Design review of the part built by this model. Coordinates are the model's own, in mm. Round coordinates to 2 decimals unless told otherwise and drop trailing zeros. Order: outer loops, then holes, each group sorted by start corner. A loop starts at its lowest first (then second) coordinate and runs counter-clockwise, first axis right, second up. Notation, with made-up numbers: M -37.5,40 L 9.5,40 A37 ccw 9.5,79 Z; hole C 20.25,38.5 d6. An arc over 180 degrees is marked long. Write item = value, one per line. Start each with the question number.
```python
from build123d import *

# Parameters (mm, degrees)
SKETCH_1_W      = 70.5
SKETCH_1_H      = 100.35
SKETCH_1_R      = 1.5
EXTRUDE_1_DEPTH = 1.6
FILLET_1_R      = 10


with BuildPart() as part:
    # 草圖1 → 填料-伸長1 (new body)
    with BuildSketch(Plane(origin=(0, 0, 0), x_dir=(1, 0, 0), z_dir=(0, 1, 0))):
        Rectangle(SKETCH_1_W, SKETCH_1_H)
        with Locations((-30, 35)):
            Circle(SKETCH_1_R, mode=Mode.SUBTRACT)
        with Locations((30, 35)):
            Circle(SKETCH_1_R, mode=Mode.SUBTRACT)
        with Locations((-30, -35)):
            Circle(SKETCH_1_R, mode=Mode.SUBTRACT)
        with Locations((30, -35)):
            Circle(SKETCH_1_R, mode=Mode.SUBTRACT)
        with BuildLine():
            Line((-25.5, 1.5), (25.5, 1.5))
            ThreePointArc((25.5, 1.5), (27, 0), (25.5, -1.5))
            Line((25.5, -1.5), (-25.5, -1.5))
            ThreePointArc((-25.5, -1.5), (-27, 0), (-25.5, 1.5))
        make_face(mode=Mode.SUBTRACT)
        with BuildLine():
            Line((1.5, 40.5), (1.5, 6.5))
            ThreePointArc((1.5, 6.5), (0, 5), (-1.5, 6.5))
            Line((-1.5, 6.5), (-1.5, 40.5))
            ThreePointArc((-1.5, 40.5), (0, 42), (1.5, 40.5))
        make_face(mode=Mode.SUBTRACT)
        with BuildLine():
            Line((1.5, -40.5), (1.5, -6.5))
            ThreePointArc((1.5, -6.5), (0, -5), (-1.5, -6.5))
            Line((-1.5, -6.5), (-1.5, -40.5))
            ThreePointArc((-1.5, -40.5), (0, -42), (1.5, -40.5))
        make_face(mode=Mode.SUBTRACT)
        with BuildLine():
            Line((13.5, 40.5), (13.5, 6.5))
            ThreePointArc((13.5, 6.5), (12, 5), (10.5, 6.5))
            Line((10.5, 6.5), (10.5, 40.5))
            ThreePointArc((10.5, 40.5), (12, 42), (13.5, 40.5))
        make_face(mode=Mode.SUBTRACT)
        with BuildLine():
            Line((13.5, -40.5), (13.5, -6.5))
            ThreePointArc((13.5, -6.5), (12, -5), (10.5, -6.5))
            Line((10.5, -6.5), (10.5, -40.5))
            ThreePointArc((10.5, -40.5), (12, -42), (13.5, -40.5))
        make_face(mode=Mode.SUBTRACT)
        with BuildLine():
            Line((25.5, 40.5), (25.5, 6.5))
            ThreePointArc((25.5, 6.5), (24, 5), (22.5, 6.5))
            Line((22.5, 6.5), (22.5, 40.5))
            ThreePointArc((22.5, 40.5), (24, 42), (25.5, 40.5))
        make_face(mode=Mode.SUBTRACT)
        with BuildLine():
            Line((25.5, -40.5), (25.5, -6.5))
            ThreePointArc((25.5, -6.5), (24, -5), (22.5, -6.5))
            Line((22.5, -6.5), (22.5, -40.5))
            ThreePointArc((22.5, -40.5), (24, -42), (25.5, -40.5))
        make_face(mode=Mode.SUBTRACT)
        with BuildLine():
            Line((-25.5, -40.5), (-25.5, -6.5))
            ThreePointArc((-25.5, -6.5), (-24, -5), (-22.5, -6.5))
            Line((-22.5, -6.5), (-22.5, -40.5))
            ThreePointArc((-22.5, -40.5), (-24, -42), (-25.5, -40.5))
        make_face(mode=Mode.SUBTRACT)
        with BuildLine():
            Line((-13.5, -40.5), (-13.5, -6.5))
            ThreePointArc((-13.5, -6.5), (-12, -5), (-10.5, -6.5))
            Line((-10.5, -6.5), (-10.5, -40.5))
            ThreePointArc((-10.5, -40.5), (-12, -42), (-13.5, -40.5))
        make_face(mode=Mode.SUBTRACT)
        with BuildLine():
            Line((-13.5, 40.5), (-13.5, 6.5))
            ThreePointArc((-13.5, 6.5), (-12, 5), (-10.5, 6.5))
            Line((-10.5, 6.5), (-10.5, 40.5))
            ThreePointArc((-10.5, 40.5), (-12, 42), (-13.5, 40.5))
        make_face(mode=Mode.SUBTRACT)
        with BuildLine():
            Line((-25.5, 40.5), (-25.5, 6.5))
            ThreePointArc((-25.5, 6.5), (-24, 5), (-22.5, 6.5))
            Line((-22.5, 6.5), (-22.5, 40.5))
            ThreePointArc((-22.5, 40.5), (-24, 42), (-25.5, 40.5))
        make_face(mode=Mode.SUBTRACT)
        with BuildLine():
            Line((-32, 41.5), (-30, 41.5))
            ThreePointArc((-30, 41.5), (-28.5, 40), (-30, 38.5))
            Line((-30, 38.5), (-32, 38.5))
            ThreePointArc((-32, 38.5), (-33.5, 40), (-32, 41.5))
        make_face(mode=Mode.SUBTRACT)
        with BuildLine():
            Line((32, 41.5), (30, 41.5))
            ThreePointArc((30, 41.5), (28.5, 40), (30, 38.5))
            Line((30, 38.5), (32, 38.5))
            ThreePointArc((32, 38.5), (33.5, 40), (32, 41.5))
        make_face(mode=Mode.SUBTRACT)
        with BuildLine():
            Line((32, -41.5), (30, -41.5))
            ThreePointArc((30, -41.5), (28.5, -40), (30, -38.5))
            Line((30, -38.5), (32, -38.5))
            ThreePointArc((32, -38.5), (33.5, -40), (32, -41.5))
        make_face(mode=Mode.SUBTRACT)
        with BuildLine():
            Line((-32, -41.5), (-30, -41.5))
            ThreePointArc((-30, -41.5), (-28.5, -40), (-30, -38.5))
            Line((-30, -38.5), (-32, -38.5))
            ThreePointArc((-32, -38.5), (-33.5, -40), (-32, -41.5))
        make_face(mode=Mode.SUBTRACT)
    extrude(amount=EXTRUDE_1_DEPTH)

    # 圓角1
    fillet_1_edges = [part.edges().sort_by_distance(p)[0] for p in [
        (35.25, 0.8, 50.175),
        (-35.25, 0.8, 50.175),
        (-35.25, 0.8, -50.175),
        (35.25, 0.8, -50.175),
    ]]
    fillet(fillet_1_edges, radius=FILLET_1_R)


solid = part.part
```
(1) Consider section A-A, the plane x = 8.5. Write out the cut boundary in (y, z) (3 decimals).
(2) Draft analysis for pull direction X (two halves, no side actions). For faces 1 (the face through (-8, 0, 10)), 2 (the face through (-32.398, 0.811, 47.168)), 3 (the face through (32.243, 0.811, -47.323)), 4 (the face through (28.8, 0.8, 35.9)), state which applies: pulls with the +X half, pulls with the -X half, needs draft (parallel to the pull), parting line crosses it, or undercut.
(3) Consider section C-C, the plane x = -12. Write out the cut boundary in (y, z) (3 decimals), then the cut area to 3 significant figures.
(4) Consider section B-B, the plane z = -37.5. Write out the cut boundary in (x, y), then the cut area to 3 significant figures.
(5) For line 1 along X through (y, z) = (1.35, 10); line 2 along X through (y, z) = (0.9, -5.5); line 3 along Z through (x, y) = (-12, 0.1) (3 decimals), list the stretches that pass through material, from the lowest coordinate up. Write a range as [from, to].
(6) Insertion check: pin 1 (0.8 mm diameter, centred on x = 30.5, y = 0.5, fed in from +Z). The pin has a flat end and moves straight along its axis. Give the tip position at first contact, or say it passes through.
(7) Consider section D-D, the plane y = 0.55. State how many separate pieces and enclosed holes the cut face has, then the cut area to 3 significant figures.
Completed:
q1.outline = M 0,-50.175 L 1.6,-50.175 L 1.6,-1.5 L 0,-1.5 Z; M 0,1.5 L 1.6,1.5 L 1.6,50.175 L 0,50.175 Z
q2.face_1 = needs draft
q2.face_2 = pulls with the -X half
q2.face_3 = pulls with the +X half
q2.face_4 = undercut
q3.outline = M 0,-50.175 L 1.6,-50.175 L 1.6,-42 L 0,-42 Z; M 0,-5 L 1.6,-5 L 1.6,-1.5 L 0,-1.5 Z; M 0,1.5 L 1.6,1.5 L 1.6,5 L 0,5 Z; M 0,42 L 1.6,42 L 1.6,50.175 L 0,50.175 Z
q3.area = 37.4 mm2
q4.outline = M -35.25,0 L -25.5,0 L -25.5,1.6 L -35.25,1.6 Z; M -22.5,0 L -13.5,0 L -13.5,1.6 L -22.5,1.6 Z; M -10.5,0 L -1.5,0 L -1.5,1.6 L -10.5,1.6 Z; M 1.5,0 L 10.5,0 L 10.5,1.6 L 1.5,1.6 Z; M 13.5,0 L 22.5,0 L 22.5,1.6 L 13.5,1.6 Z; M 25.5,0 L 35.25,0 L 35.25,1.6 L 25.5,1.6 Z
q4.area = 88.8 mm2
q5.line_1 = [-35.25, -25.5], [-22.5, -13.5], [-10.5, -1.5], [1.5, 10.5], [13.5, 22.5], [25.5, 35.25]
q5.line_2 = [-35.25, -25.12], [-22.88, -13.12], [-10.88, -1.12], [1.12, 10.88], [13.12, 22.88], [25.12, 35.25]
q5.line_3 = [-50.175, -42], [-5, -1.5], [1.5, 5], [42, 50.175]
q6.pin_1 = 48.92
q7.separate_pieces = 1
q7.enclosed_holes = 19
q7.area = 5,660 mm2
